from build123d import *

# Parameters (mm, degrees)
SKETCH1_R           = 12.5
BOSS_EXTRUDE1_DEPTH = 14.7
SHELL1_T            = -1
SKETCH2_W           = 15
SKETCH2_H           = 2.2
CUT_EXTRUDE1_DEPTH  = 24.7


with BuildPart() as part:
    # Sketch1 → Boss-Extrude1 (new body)
    with BuildSketch(Plane(origin=(0, 0, 0), x_dir=(1, 0, 0), z_dir=(0, 1, 0))):
        with Locations(Location((0, 0, 0), (0, 0, 270))):
            Circle(SKETCH1_R)
    extrude(amount=BOSS_EXTRUDE1_DEPTH)

    # Shell1
    shell1_openings = [part.faces().sort_by_distance(p)[0] for p in [
        (0, 14.7, 0),
    ]]
    offset(amount=SHELL1_T, openings=shell1_openings, kind=Kind.INTERSECTION)

    # Sketch2 → Cut-Extrude1 (cut)
    with BuildSketch(Plane(origin=(0, 0, 0), x_dir=(0, 0, -1), z_dir=(1, 0, 0))):
        with Locations((0, 11.1)):
            Rectangle(SKETCH2_W, SKETCH2_H)
    extrude(amount=CUT_EXTRUDE1_DEPTH, mode=Mode.SUBTRACT)


solid = part.part
Input: part model. Units: mm. Frame: model coordinates. A direction names the side the tool comes from. Coordinates: 2 decimals unless noted, no trailing zeros. Loops run counter-clockwise (first coordinate to the right, second up) from the corner with the lowest first, then second, coordinate; pieces in that order, holes last.
Q1. Material intervals for line 1 (Z direction, x = 0.25, y = 6.5); line 2 (Y direction, x = 0.5, z = -8.5); line 3 (X direction, y = 11.5, z = 0), sorted ascending.
Q2. Set-up query: faces 5 (the face through (12, 10, 0)), 6 (the face through (-12.203, 7.247, -2.71)), 7 (the face through (-11.227, 7.754, -2.493)). Return all of +Z, -Z, +X, -X, +Y, -Y with unobstructed straight access to the full face (end or side cutting, diameter ignored); none if empty.
Q3. Cut plane B-B (x = 0). Output: boundary loops of the cut face in (y, z).
Q4. Cut plane C-C (y = 11.25). Output: boundary loops of the cut face in (x, z).
Q5. Cut plane D-D (z = 10). Output: boundary loops of the cut face in (x, y), then the cut area to 3 significant figures.
Q6. Cut plane A-A (z = 0). Output: boundary loops of the cut face in (x, y), then the cut area to 3 significant figures.
Q7. Draft query along Y for faces 1 (the face through (9, 11, 7.5)), 2 (the face through (0, 0, 0)), 3 (the face through (9, 11, -7.5)), 4 (the face through (0, 1, 0)). Return one class per face: +Y half, -Y half, draft (parallel to the pull), parting line (faces both ways), or undercut.
Q8. Contact query for flat-ended pins moving along their axis: pin 1 (2 mm diameter, centred on y = 5.5, z = -4.5, fed in from -X); pin 2 (1.5 mm diameter, centred on x = 0, z = -8, fed in from +Y); pin 3 (6 mm diameter, centred on x = 7, y = 4, fed in from -Z). Output: stop coordinate, or through.
Working result:
1. line 1: z = -12.5 to -11.5, 11.5 to 12.5
1. line 2: y = 0 to 1
1. line 3: x = -12.5 to -11.5
2. face 5: +X
2. face 6: +Y, -Y
2. face 7: +Y
3. outline: (0, -12.5) - (14.7, -12.5) - (14.7, -11.5) - (1, -11.5) - (1, 11.5) - (14.7, 11.5) - (14.7, 12.5) - (0, 12.5) - close
4. outline: (8.72, -7.5) arc R11.5 cw (long way) to (8.72, 7.5) - (10, 7.5) arc R12.5 ccw (long way) to (10, -7.5) - close
5. outline: (-7.5, 0) - (7.5, 0) - (7.5, 14.7) - (5.68, 14.7) - (5.68, 1) - (-5.68, 1) - (-5.68, 14.7) - (-7.5, 14.7) - close
5. area: 64.9 mm2
6. outline: (-12.5, 0) - (12.5, 0) - (12.5, 10) - (11.5, 10) - (11.5, 1) - (-11.5, 1) - (-11.5, 14.7) - (-12.5, 14.7) - close; (11.5, 12.2) - (12.5, 12.2) - (12.5, 14.7) - (11.5, 14.7) - close
6. area: 50.2 mm2
7. face 1: undercut
7. face 2: -Y half
7. face 3: undercut
7. face 4: +Y half
8. pin 1: stops at x = -12
8. pin 2: stops at y = 1
8. pin 3: stops at z = -11.84
